Input: dimensioned drawing with shaded views. Units: mm. Origin: part minimum x, y, z. Round coordinates to 2 decimals unless told otherwise and drop trailing zeros. Loops run counter-clockwise (first coordinate to the right, second up) from the corner with the lowest first, then second, coordinate; pieces in that order, holes last. Notation, with made-up numbers: (89.5, 76) -> (120.5, 76) arc R28 ccw to (120.5, 96) -> close; hole circle Ø8 at (-4, 6). An arc over 180 degrees is marked (long way). Answer as a JSON object with one key per item and string values.
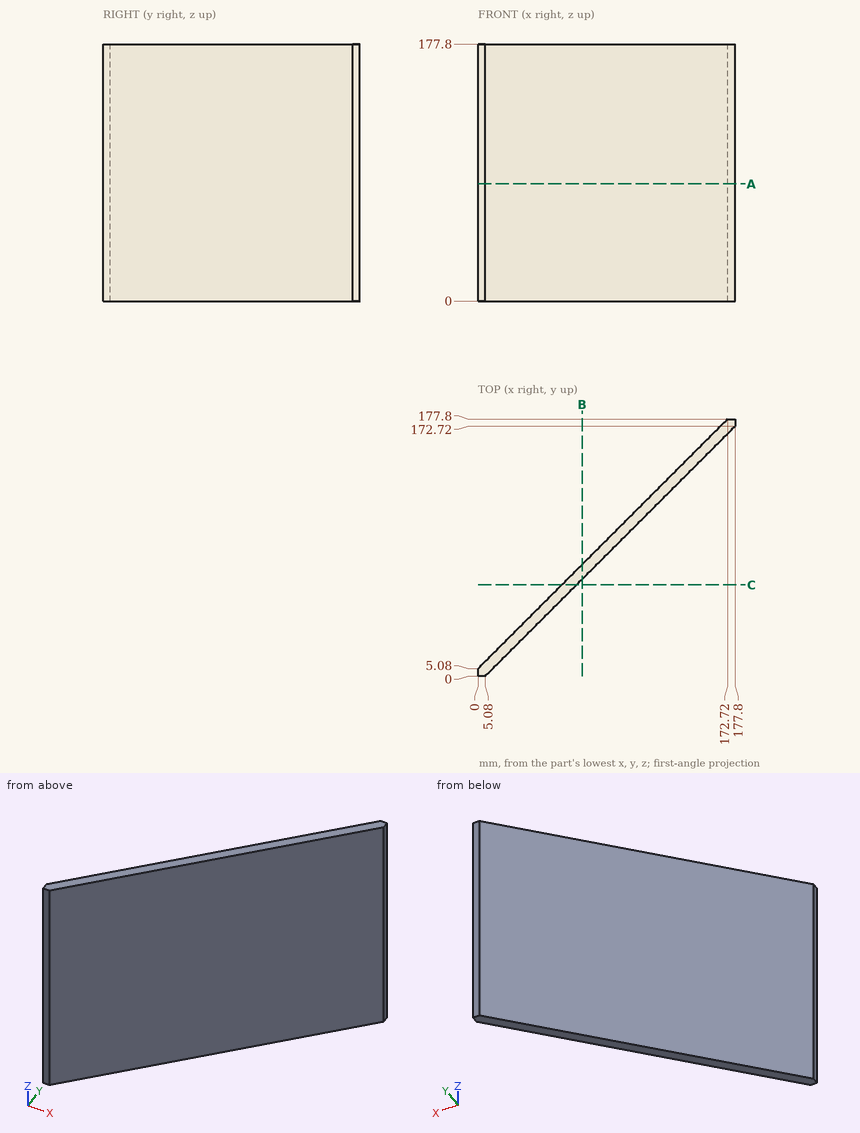
1) Section A-A, the plane z = 81. Output: boundary loops of the cut face in (x, y), plus the area to 3 significant figures.
Output:
{"outline": "(0, 0) -> (5.08, 0) -> (177.8, 172.72) -> (177.8, 177.8) -> (172.72, 177.8) -> (0, 5.08) -> close", "area": "1,780 mm^2"}
2) Section B-B, the plane x = 72. Output: boundary loops of the cut face in (y, z).
Output:
{"outline": "(66.92, 0) -> (77.08, 0) -> (77.08, 177.8) -> (66.92, 177.8) -> close"}
3) Contact query for flat-ended pins moving along their axis: P1, Ø8, axis at y = 141, z = 117, coming from the -X side; P2, Ø1, axis at y = 147, z = 136, coming from the +X side; P3, Ø10, axis at x = 95.5, z = 110.5, coming from the -Y side. Output: stop coordinate, or through.
Output:
{"P1": "stops at x = 131.92", "P2": "stops at x = 152.58", "P3": "stops at y = 85.42"}
4) Section C-C, the plane y = 63. Output: boundary loops of the cut face in (x, z).
Output:
{"outline": "(57.92, 0) -> (68.08, 0) -> (68.08, 177.8) -> (57.92, 177.8) -> close"}
5) Ray query, probe 1 along Y at (x, z) = (107, 59.5); probe 2 along X at (y, z) = (66.5, 145.5); probe 3 along X at (y, z) = (35, 53.5). Return the intervals inside material, ascending.
Output:
{"probe 1": "y = 101.92 to 112.08", "probe 2": "x = 61.42 to 71.58", "probe 3": "x = 29.92 to 40.08"}
